Read the model definition and answer for the solid it produces. Units are mm, in the model's axes. A direction names the side the tool comes from. Give positions to 0.01 mm unless a question says otherwise; leave off trailing zeros. Write each loop counter-clockwise with the first axis right and the second up, starting at its lowest first coordinate (ties: lowest second). Pieces come first, ordered by that corner, then holes. Notation, with made-up numbers: M 82,85.25 L 99,85.25 A37 ccw 99,123.25 Z; hole C -12.5,62 d11. An arc over 180 degrees is marked long. Answer as CSV lines item,"result". Start each with the question number.
```python
from build123d import *

# Parameters (mm, degrees)
SKETCH1_R           = 6.1
SKETCH1_R_2         = 1.5
BOSS_EXTRUDE1_DEPTH = 2.3
SKETCH2_R           = 4.4
SKETCH2_R_2         = 3
BOSS_EXTRUDE2_DEPTH = 3.2
SKETCH3_R           = 0.75
BOSS_EXTRUDE3_DEPTH = 2.3
CIRPATTERN1_COUNT   = 4


with BuildPart() as part:
    # Sketch1 → Boss-Extrude1 (new body)
    with BuildSketch(Plane(origin=(0, 0, 0), x_dir=(1, 0, 0), z_dir=(0, 1, 0))):
        Circle(SKETCH1_R)
        Circle(SKETCH1_R_2, mode=Mode.SUBTRACT)
    extrude(amount=BOSS_EXTRUDE1_DEPTH)

    # Sketch2 → Boss-Extrude2 (add)
    with BuildSketch(Plane(origin=(0, 2.3, 0), x_dir=(1, 0, 0), z_dir=(0, 1, 0))):
        Circle(SKETCH2_R)
        Circle(SKETCH2_R_2, mode=Mode.SUBTRACT)
    extrude(amount=BOSS_EXTRUDE2_DEPTH)

    # Sketch3 → Boss-Extrude3 (add)
    with BuildSketch(Plane.XZ):
        with BuildLine():
            Line((-4.5, -4.118252056), (-2.468988638, -16.892549493))
            ThreePointArc((-2.468988638, -16.892549493), (0, -19), (2.468988638, -16.892549493))
            Line((2.468988638, -16.892549493), (4.5, -4.118252056))
            ThreePointArc((4.5, -4.118252056), (0, -6.1), (-4.5, -4.118252056))
        make_face()
        with Locations((0, -16)):
            Circle(SKETCH3_R, mode=Mode.SUBTRACT)
        with Locations((0, -13)):
            Circle(SKETCH3_R, mode=Mode.SUBTRACT)
        with Locations((0, -10)):
            Circle(SKETCH3_R, mode=Mode.SUBTRACT)
        with Locations((0, -7)):
            Circle(SKETCH3_R, mode=Mode.SUBTRACT)
    boss_extrude3 = extrude(amount=-BOSS_EXTRUDE3_DEPTH)

    # CirPattern1: Boss-Extrude3 ×4 about axis
    cirpattern1_axis = Axis((0, 0, 0), (0, 1, 0))
    for i in range(1, CIRPATTERN1_COUNT):
        add(boss_extrude3.rotate(cirpattern1_axis, i * 360 / CIRPATTERN1_COUNT))


solid = part.part
```
1. For faces 1 (the face through (-1.5, 2.3, -4.3)), 2 (the face through (-12.256, 1.134, 0.098)), determine the directions among +Z, -Z, +X, -X, +Y, -Y from which every point of the face is accessible in a straight line to the end or side of a thin tool.
2. Find the intervals of material crossed by line 1 (Z direction, x = 7.5, y = 2.1); line 2 (X direction, y = 3.9, z = 2.5); line 3 (Y direction, x = 9, z = 1), in increasing order. Write a range as [from, to].
3. Find section B-B on z = 10. Determine the outline of the cut face in (x, y), then the cut area to 3 significant figures.
4. Given pin 1 (1.7 mm diameter, centred on x = 10, z = 0, fed in from +Y); pin 2 (1.5 mm diameter, centred on x = 6.5, z = 4, fed in from -Y); pin 3 (1.4 mm diameter, centred on x = 0, z = 7, fed in from -Y), each flat-ended and moving along its own axis, determine where each tip first touches the part or whether it passes through.
5. Find section A-A on y = 1.6. State how many separate pieces and enclosed holes the cut face has, then the cut area to 3 significant figures.
6. Find section D-D on x = 16. Determine the outline of the cut face in (y, z).
7. Determine the mould class of faces 3 (the face through (19, 1, 0)), 4 (the face through (-10.757, 1.134, -3.444)), 5 (the face through (-0.163, 1.134, -7.732)) for opening direction X: +X half, -X half, draft (parallel to the pull), parting line (faces both ways), or undercut.
Computed:
1,face 1,"+Y"
1,face 2,"+Y, -Y"
2,line 1,"z = [-3.96, -0.56], [0.56, 3.96]"
2,line 2,"x = [-3.62, -1.66], [1.66, 3.62]"
2,line 3,"y = [0, 2.3]"
3,outline,"M -3.56,0 L -0.75,0 L -0.75,2.3 L -3.56,2.3 Z; M 0.75,0 L 3.56,0 L 3.56,2.3 L 0.75,2.3 Z"
3,area,"12.9 mm^2"
4,pin 1,"stops at y = 2.3"
4,pin 2,"stops at y = 0"
4,pin 3,"passes through"
5,separate pieces,"1"
5,enclosed holes,"17"
5,area,"420 mm^2"
6,outline,"M 0,-2.61 L 2.3,-2.61 L 2.3,-0.75 L 0,-0.75 Z; M 0,0.75 L 2.3,0.75 L 2.3,2.61 L 0,2.61 Z"
7,face 3,"+X half"
7,face 4,"-X half"
7,face 5,"undercut"
